```python
from build123d import *
from OCP.BRepAlgoAPI import BRepAlgoAPI_Cut
from OCP.TopTools import TopTools_ListOfShape

# Parameters (mm, degrees)
SKETCH1_W           = 296
SKETCH1_H           = 190
SKETCH1_R           = 6
SKETCH1_R_2         = 2.5
SKETCH1_W_2         = 12
SKETCH1_H_2         = 19
BOSS_EXTRUDE1_DEPTH = 12
CUT_EXTRUDE2_START  = 104.787049
SKETCH3_R           = 1.5
CUT_EXTRUDE2_DEPTH  = 20
CUT_EXTRUDE3_START  = -171.212951
SKETCH3_2_R         = 1.5
CUT_EXTRUDE3_DEPTH  = 20
CUT_EXTRUDE4_START  = 12
SKETCH4_R           = 4
CUT_EXTRUDE4_DEPTH  = 4


with BuildPart() as part:
    # Sketch1 → Boss-Extrude1 (new body)
    with BuildSketch(Plane(origin=(0, 0, 0), x_dir=(1, 0, 0), z_dir=(0, 1, 0))):
        with Locations((-43.212950637, 23.312387878)):
            Rectangle(SKETCH1_W, SKETCH1_H)
        with Locations(Location((83.787049363, 58.312387878, 0), (0, 0, 270))):
            Circle(SKETCH1_R, mode=Mode.SUBTRACT)
        with Locations(Location((89.787049363, 103.312387878, 0), (0, 0, 270))):
            Circle(SKETCH1_R_2, mode=Mode.SUBTRACT)
        with Locations(Location((77.787049363, 103.312387878, 0), (0, 0, 270))):
            Circle(SKETCH1_R_2, mode=Mode.SUBTRACT)
        with Locations((83.787049363, 83.812387878)):
            Rectangle(SKETCH1_W_2, SKETCH1_H_2, mode=Mode.SUBTRACT)
    extrude(amount=BOSS_EXTRUDE1_DEPTH)


with BuildPart() as cut_extrude2_tool:
    # Sketch3 → Cut-Extrude2 (new body)
    with BuildSketch(Plane(origin=(0, 0, 0), x_dir=(0, 0, -1), z_dir=(1, 0, 0)).offset(CUT_EXTRUDE2_START)):
        with Locations(Location((98.312387878, 6, 0), (0, 0, 180))):
            Circle(SKETCH3_R)
        with Locations(Location((-29.687612122, 6, 0), (0, 0, 180))):
            Circle(SKETCH3_R)
    extrude(amount=-CUT_EXTRUDE2_DEPTH)


with BuildPart() as part_1:
    add(part.part)

    # Cut-Extrude2: cut by cut_extrude2_tool, with a tolerance
    cut_extrude2_stock = TopTools_ListOfShape()
    cut_extrude2_stock.Append(part_1.part.wrapped)
    cut_extrude2_tools = TopTools_ListOfShape()
    cut_extrude2_tools.Append(cut_extrude2_tool.part.wrapped)
    cut_extrude2_cut = BRepAlgoAPI_Cut()
    cut_extrude2_cut.SetArguments(cut_extrude2_stock)
    cut_extrude2_cut.SetTools(cut_extrude2_tools)
    cut_extrude2_cut.SetFuzzyValue(0.00001)
    cut_extrude2_cut.Build()
    add(Compound.cast(cut_extrude2_cut.Shape()).solids(), mode=Mode.REPLACE)

    # Sketch3<2> → Cut-Extrude3 (cut)
    with BuildSketch(Plane(origin=(0, 0, 0), x_dir=(0, 0, -1), z_dir=(1, 0, 0)).offset(CUT_EXTRUDE3_START)):
        with Locations(Location((98.312387878, 6, 0), (0, 0, 180))):
            Circle(SKETCH3_2_R)
        with Locations(Location((-29.687612122, 6, 0), (0, 0, 180))):
            Circle(SKETCH3_2_R)
    extrude(amount=-CUT_EXTRUDE3_DEPTH, mode=Mode.SUBTRACT)

    # Sketch4 → Cut-Extrude4 (cut)
    with BuildSketch(Plane(origin=(0, 0, 0), x_dir=(1, 0, 0), z_dir=(0, 1, 0)).offset(CUT_EXTRUDE4_START)):
        with Locations(Location((89.787049363, 103.312387878, 0), (0, 0, 270))):
            Circle(SKETCH4_R)
        with Locations(Location((77.787049363, 103.312387878, 0), (0, 0, 270))):
            Circle(SKETCH4_R)
    extrude(amount=-CUT_EXTRUDE4_DEPTH, mode=Mode.SUBTRACT)


solid = part_1.part
```
Verification items for the finished model (mm, model axes). A direction names the side the tool comes from. Coordinates: 2 decimals unless noted, no trailing zeros. Order: outer loops, then holes, each group sorted by start corner. A loop starts at its lowest first (then second) coordinate and runs counter-clockwise, first axis right, second up. Notation, with made-up numbers: (-37, 45) -> (-12, 45) arc R24 cw to (-12, 72) -> close; hole circle Ø7 at (14, -37). An arc over 180 degrees is marked (long way). Answer as CSV lines item,"result". Start each with the question number.
1) Release check for a two-part mould opening along X. For faces 4 (the face through (-45, 0, -25)), 5 (the face through (87, 8, -103)), 6 (the face through (104.787, 6, -22)) record: released by +X, released by -X, zero draft, split by the parting line, or undercut.
2) Set-up check for faces 1 (the face through (89.787, 6, -84)), 2 (the face through (-191.213, 6, -22)), 3 (the face through (85.882, 10.028, -104.18)): record each of +Z, -Z, +X, -X, +Y, -Y from which the full face is reachable in a straight line by a thin tool's end or side.
3) Material ranges on L1, parallel to Z at x = 96.5, y = 6; L2, parallel to Z at x = 92, y = 5.5; L3, parallel to X at y = 4.25, z = -91, recorded low to high. Write a range as [from, to].
4) Cross-section at A-A, the plane z = -81.5. Record the boundary of the cut face in (x, y), then the cut area to 3 significant figures.
5) Gauge pin test, flat ends, axial feed: pin 1 Ø1.8 at (y, z) = (6, -98.31) entering from -X; pin 2 Ø2.5 at (y, z) = (6, 29.69) entering from +X; pin 3 Ø2.5 at (x, z) = (91, -101.5) entering from +Y. Record the tip position at first contact, or that the pin passes through.
Conclusion:
1,face 4,"zero draft"
1,face 5,"undercut"
1,face 6,"released by +X"
2,face 1,"+Y, -Y"
2,face 2,"+Z, -Z, -X, +Y, -Y"
2,face 3,"+Y"
3,L1,"z = [-118.31, -99.81], [-96.81, 28.19], [31.19, 71.69]"
3,L2,"z = [-118.31, -104.48], [-102.15, -99.73], [-96.9, 28.27], [31.1, 71.69]"
3,L3,"x = [-191.21, 77.79], [89.79, 104.79]"
4,outline,"(-191.21, 0) -> (77.79, 0) -> (77.79, 12) -> (-191.21, 12) -> close; (89.79, 0) -> (104.79, 0) -> (104.79, 12) -> (89.79, 12) -> close"
4,area,"3,410 mm²"
5,pin 1,"stops at x = -171.21"
5,pin 2,"stops at x = 84.79"
5,pin 3,"stops at y = 8"
